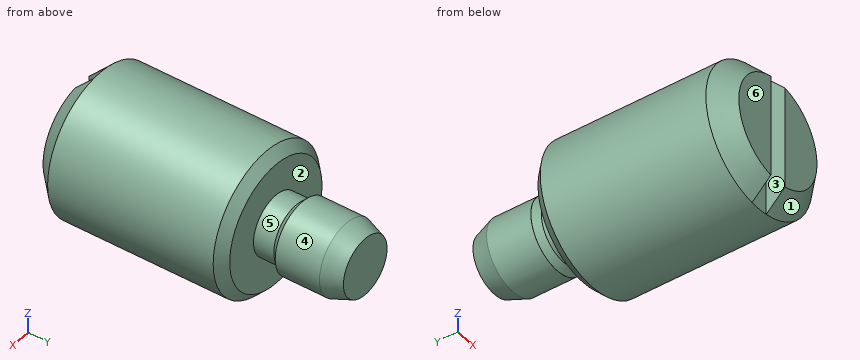
Autodesk Inventor part; units mm, degrees
ref_plane "YZ Plane" through (0, 0, 0) normal (1, 0, 0) x (0, 1, 0)
ref_plane "XZ Plane" through (0, 0, 0) normal (0, 1, 0) x (-1, 0, 0)
ref_plane "XY Plane" through (0, 0, 0) normal (0, 0, 1) x (1, 0, 0)
sketch "Sketch1" plane through (0, 0, 0) normal (0, 1, 0) x (-1, 0, 0)
  circle A0 centre (0, 0) radius 4.7625
  line L0 (0.635, 4.7625) -> (-0.635, 4.7625)
  line L1 (-0.635, 4.7625) -> (-0.635, -4.7625)
  line L2 (-0.635, -4.7625) -> (0.635, -4.7625)
  line L3 (0.635, -4.7625) -> (0.635, 4.7625)
  line L4 (0.635, 4.7625) -> (-0.635, -4.7625) construction
  line L5 (-0.635, 4.7625) -> (0.635, -4.7625) construction
  point P0 (0.635, -4.72)
  point P1 (0.635, 4.72)
  point P2 (-0.635, 4.72)
  point P3 (-0.635, -4.72)
  dimension "d0" = 9.525
  dimension "d9" = 1.27
extrude "Extrusion1" add sketch "Sketch1" along normal blind 13.081 contours A0 L3 | L3 A0 L1 | L1 A0
sketch "Sketch2" plane through (0, 13.081, 0) normal (0, 1, 0) x (1, 0, 0)
  circle A0 centre (0, 0) radius 2.0003
  dimension "d3" = 4.0005
extrude "Extrusion2" add sketch "Sketch2" along normal blind 1.778
sketch "Sketch3" plane through (0, 14.859, 0) normal (0, 1, 0) x (1, 0, 0)
  circle A0 centre (0, 0) radius 2.413
  dimension "d19" = 4.826
extrude "Extrusion4" add sketch "Sketch3" along normal blind 4.2545
extrude "Extrusion3" cut sketch "Sketch1" along normal blind 1.27 contours L3 A0 L1
chamfer "Chamfer2" distance 0.635 angle 45 1 edges at (4.7625, 13.081, 0)
chamfer "Chamfer1" distance 1.27 angle 45 3 edges at (-3.5851, 0, -3.1351) (-3.5851, 0, 3.1351) (4.7625, 0, 0)
chamfer "Chamfer3" distance 0.4064 angle 45 1 edges at (-2.0003, 14.859, 0)
chamfer "Chamfer4" distance 1.27 angle 20 1 edges at (-2.413, 19.1135, 0) measured on face at (2.4052, 17.6953, 0.1942)
thread "Thread3"
properties part number "0.375 Shaft" material "Stainless Steel"
Check sheet for the modelled part. Datum: model origin and axes. Units: mm. Face numbers are marked on the shaded views. A direction names the side the tool comes from. Round coordinates to 2 decimals unless told otherwise and drop trailing zeros. Write each loop counter-clockwise with the first axis right and the second up, starting at its lowest first coordinate (ties: lowest second). Pieces come first, ordered by that corner, then holes. Notation, with made-up numbers: (55, 68.25) -> (98, 68.25) arc R17 ccw to (98, 91.25) -> close; hole circle Ø2 at (-39.75, -24). An arc over 180 degrees is marked (long way). Put each result on its own line as item: value.
(1) Mould release check, pull along Y, two halves, no side actions. Record for the marked faces 4, 5 and 6: released by +Y, released by -Y, zero draft, split by the parting line, or undercut.
Values found:
face 4: zero draft
face 5: undercut
face 6: released by -Y
(2) Go/stop test with a flat-tipped pin: pin 1 Ø3 at (y, z) = (12.5, -2.5) entering from +X. Record where the tip stops, or that it passes through.
Values found:
pin 1: stops at x = 4.66
(3) Sectioned sample at D-D (y = 16.25). Enter the section's corners in (x, z).
Values found:
outline: circle Ø4.83 at (0, 0)
(4) Tool access check on the marked faces 1, 2 and 3. Record the directions out of +Z, -Z, +X, -X, +Y, -Y that give a thin tool (end or side, any length) a straight path to the whole face; none if there is none.
Values found:
face 1: +X, -Y
face 2: none
face 3: +Z, -Z, -Y
(5) Material ranges on line 1 (Y direction, x = -3.25, z = 0.25); line 2 (X direction, y = 1, z = 1) (3 decimals); line 3 (X direction, y = 10.5, z = 1.75), recorded low to high.
Values found:
line 1: y = 0 to 13.08
line 2: x = -4.38 to -0.635, 0.635 to 4.38
line 3: x = -4.43 to 4.43
(6) Sectioned sample at C-C (y = 1.5). Enter the section's corners in (x, z) (1 decimal), plus the area to 3 significant figures.
Values found:
outline: circle Ø9.5 at (0, 0)
area: 71.3 mm^2
